Study the drawing (mm; zero at the part's minimum x, y, z) and answer. Coordinates: 2 decimals unless noted, no trailing zeros. Order: outer loops, then holes, each group sorted by start corner. A loop starts at its lowest first (then second) coordinate and runs counter-clockwise, first axis right, second up.
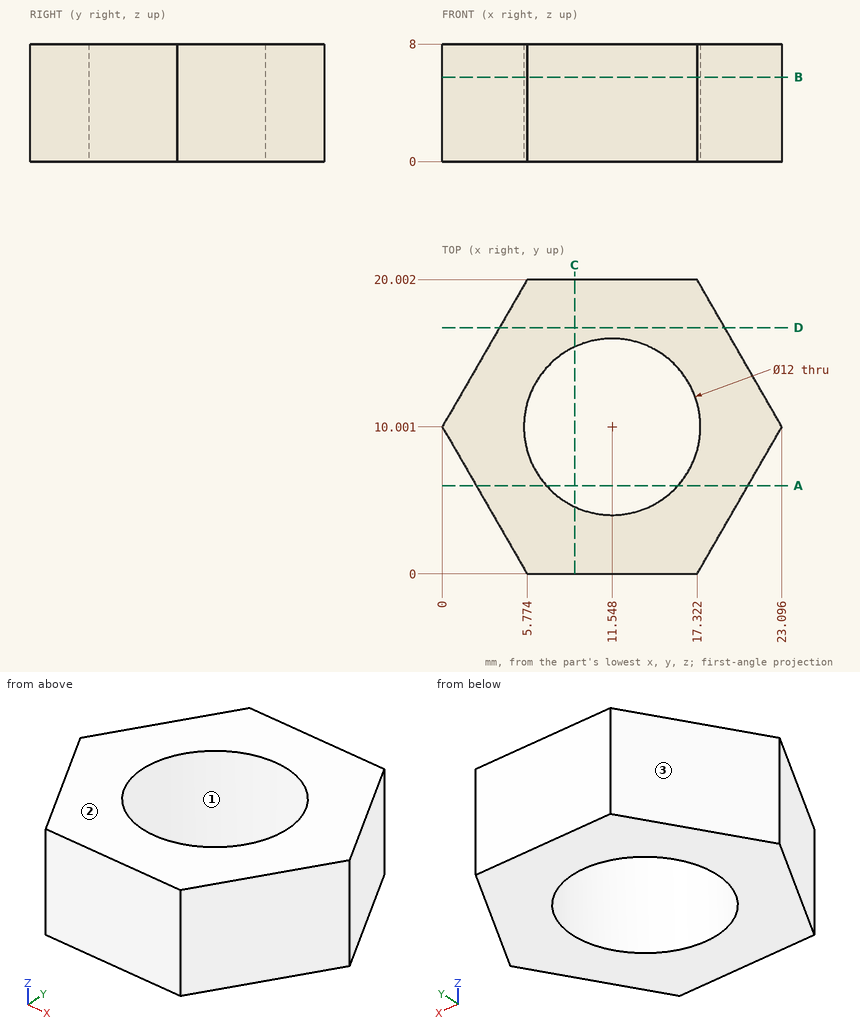
(1) Given pin 1 Ø2 at (x, y) = (11.5, 6.5) entering from +Z; pin 2 Ø1.5 at (x, z) = (20, 7) entering from -Y; pin 3 Ø4 at (x, z) = (12.5, 1.5) entering from -Y, each flat-ended and moving along its own axis, determine where each tip first touches the part or whether it passes through.
(2) Find section D-D on y = 16.75. Determine the outline of the cut face in (x, z).
(3) Find section B-B on z = 5.75. Determine the outline of the cut face in (x, y), then the cut area to 3 significant figures.
(4) Find section C-C on x = 9. Determine the outline of the cut face in (y, z), then the cut area to 3 significant figures.
(5) Find the intervals of material crossed by probe 1 along Y at (x, z) = (10.5, 1.25); probe 2 along X at (y, z) = (8.5, 5.5) (1 decimal); probe 3 along X at (y, z) = (15, 6.5) (1 decimal), in increasing order.
(6) The mould has two halves that part along Y. Classify the marked faces 1, 2 and 3: pulls with the +Y half, pulls with the -Y half, needs draft (parallel to the pull), parting line crosses it, or undercut.
(7) Find section A-A on y = 6. Determine the outline of the cut face in (x, z).
Resolved:
1. pin 1: passes through
1. pin 2: stops at y = 3.34
1. pin 3: stops at y = 0
2. outline: (3.9, 0) - (19.2, 0) - (19.2, 8) - (3.9, 8) - close
3. outline: (0, 10) - (5.77, 0) - (17.32, 0) - (23.1, 10) - (17.32, 20) - (5.77, 20) - close; hole circle Ø12 at (11.55, 10)
3. area: 233 mm2
4. outline: (0, 0) - (4.57, 0) - (4.57, 8) - (0, 8) - close; (15.43, 0) - (20, 0) - (20, 8) - (15.43, 8) - close
4. area: 73.1 mm2
5. probe 1: y = 0 to 4.09, 15.91 to 20
5. probe 2: x = 0.9 to 5.7, 17.4 to 22.2
5. probe 3: x = 2.9 to 8.2, 14.9 to 20.2
6. face 1: undercut
6. face 2: needs draft
6. face 3: pulls with the +Y half
7. outline: (2.31, 0) - (7.08, 0) - (7.08, 8) - (2.31, 8) - close; (16.02, 0) - (20.79, 0) - (20.79, 8) - (16.02, 8) - close
